```python
from build123d import *

# Parameters (mm, degrees)
F1_DEPTH = 7
F2_R     = 1.2


# Not quite as in the source:
# - a feature names something its author has since deleted; it is built from what else it names


with BuildPart() as f1:
    # F0 (on Top) → F1 (new body)
    with BuildSketch(Plane.XY):
        with BuildLine():
            Line((-5, -5), (0, -5))
            ThreePointArc((0, -5), (-3.5355339059, -3.5355339059), (-5, 0))
            Line((-5, 0), (-5, -5))
        make_face()
        with BuildLine():
            ThreePointArc((0, -5), (3.5355339059, -3.5355339059), (5, 0))
            ThreePointArc((5, 0), (3.5355339059, 3.5355339059), (0, 5))
            Line((0, 5), (0, 2))
            ThreePointArc((0, 2), (1.4142135624, 1.4142135624), (2, 0))
            ThreePointArc((2, 0), (0.2572150448, -1.9833911416), (-1.9338404207, -0.5101580414))
            Line((-1.9338404207, -0.5101580414), (-3.1027593412, 3.9208270136))
            ThreePointArc((-3.1027593412, 3.9208270136), (-4.5007664184, 2.177866306), (-5, 0))
            ThreePointArc((-5, 0), (-3.5355339059, -3.5355339059), (0, -5))
        make_face()
        with BuildLine():
            ThreePointArc((-5, 0), (-4.5007664184, 2.177866306), (-3.1027593412, 3.9208270136))
            Line((-3.1027593412, 3.9208270136), (-3.3874512792, 5))
            Line((-3.3874512792, 5), (-5, 5))
            Line((-5, 5), (-5, 0))
        make_face()
    extrude(amount=F1_DEPTH)

    # F2
    f2_edges = [f1.edges().sort_by_distance(p)[0] for p in [
        (1.584348, -1.220591, 0),
        (1.584348, -1.220591, 7),
        (5, 0, 0),
        (5, 0, 7),
        (0, 5, 3.5),
        (0, 2, 3.5),
        (0, 3.5, 7),
        (0, 3.5, 0),
        (-3.387451, 5, 3.5),
        (-2.5, -5, 0),
        (-2.5, -5, 7),
        (-2.660646, 2.244921, 0),
        (-2.660646, 2.244921, 7),
    ]]
    fillet(f2_edges, radius=F2_R)


solid = f1.part
```
Can you work these out from the model? Positions are in its coordinate system, mm. A direction names the side the tool comes from. Round coordinates to 2 decimals unless told otherwise and drop trailing zeros. Loops run counter-clockwise (first coordinate to the right, second up) from the corner with the lowest first, then second, coordinate; pieces in that order, holes last.
Item 1: If we mould it in two halves opening along Y, with no side actions, what happens to faces 1 (the cylindrical face through (-3.571, 4.744, 3.548)), 2 (the flat face through (-3, -5, 3)), 3 (the cylindrical face through (0.2, 2.3, 3.5))? For each: +Y half, -Y half, draft (parallel to the pull), parting line (faces both ways), or undercut.
Item 2: Suppose I cut it at A-A, the plane z = 2.75. Write out the boundary of the cut face in (x, y).
Item 3: Which directions (+Z, -Z, +X, -X, +Y, -Y) give clear straight access to the entire face, cutting with the end or side of a thin tool? Please do faces 4 (the cylindrical face through (-2.465, -4.658, 6.639)), 5 (the cylindrical face through (0.342, 3.282, 6.639)), 6 (the cylindrical face through (0.342, 3.282, 0.361)).
Item 4: Will these pins go through, and if not, where does the flat tip stop? pin 1 Ø4 at (x, y) = (2, -3.5) entering from +Z; pin 2 Ø2 at (x, z) = (-2.5, 1) entering from +Y; pin 3 Ø1 at (x, y) = (2, 0.5) entering from -Z; pin 4 Ø2 at (x, z) = (3.5, 2) entering from -Y.
Item 5: Suppose I cut it at B-B, the plane z = 0.5. Write out the boundary of the cut face in (x, y).
Item 6: Please list where these lines run through material, in increasing order: L1, parallel to X at y = 0.5, z = 5; L2, parallel to Y at x = 1.5, z = 2.75; L3, parallel to X at y = 2.5, z = 5.5.
Reported:
1. face 1: +Y half
1. face 2: -Y half
1. face 3: undercut
2. outline: (-5, -5) - (0, -5) arc R5 ccw to (1.58, 4.74) arc R1.2 ccw to (0, 3.61) - (0, 2.97) arc R1.2 ccw to (0.75, 1.85) arc R2 cw (long way) to (-1.93, -0.51) - (-3.15, 4.11) arc R1.2 ccw to (-4.31, 5) - (-5, 5) - close
3. face 4: +Z, +X, -X, -Y
3. face 5: +Z, +Y
3. face 6: -Z, +Y
4. pin 1: stops at z = 7
4. pin 2: stops at y = 4.68
4. pin 3: stops at z = 0.18
4. pin 4: stops at y = -4.33
5. outline: (-5, -4.77) - (0, -4.77) arc R4.77 ccw to (1.51, 4.53) arc R0.97 ccw to (0.23, 3.61) - (0.23, 2.97) arc R0.97 ccw to (0.83, 2.06) arc R2.23 cw (long way) to (-2.15, -0.57) - (-3.55, 4.73) arc R1.2 ccw to (-4.31, 5) - (-5, 5) - close
6. L1: x = -5 to -2.2, 1.94 to 4.97
6. L2: y = -4.77 to -1.32, 1.32 to 4.77
6. L3: x = -5 to -2.73, 0.09 to 4.33
